from build123d import *

# Parameters (mm, degrees)
SKETCH2_W            = 125
SKETCH2_H            = 85
CREATE_BEAM_DEPTH    = 40
SKETCH3_W            = 119
SKETCH3_H            = 79
SKETCH3_R            = 7
REMOVE_OUTSIDE_DEPTH = 35
SKETCH4_R            = 7
LOWER_PILLARS_DEPTH  = 20


with BuildPart() as part:
    # Sketch2 → Create Beam (new body)
    with BuildSketch(Plane(origin=(0, 0, 0), x_dir=(1, 0, 0), z_dir=(0, 1, 0))):
        with Locations((62.5, 42.5)):
            Rectangle(SKETCH2_W, SKETCH2_H)
    extrude(amount=CREATE_BEAM_DEPTH)

    # Sketch3 → Remove Outside (cut)
    with BuildSketch(Plane(origin=(0, 40, 0), x_dir=(1, 0, 0), z_dir=(0, 1, 0))):
        with Locations((62.5, 42.5)):
            Rectangle(SKETCH3_W, SKETCH3_H)
        with Locations(Location((91, 33, 0), (0, 0, 270))):
            Circle(SKETCH3_R, mode=Mode.SUBTRACT)
        with Locations(Location((72, 33, 0), (0, 0, 270))):
            Circle(SKETCH3_R, mode=Mode.SUBTRACT)
        with Locations(Location((53, 33, 0), (0, 0, 270))):
            Circle(SKETCH3_R, mode=Mode.SUBTRACT)
        with Locations(Location((34, 33, 0), (0, 0, 270))):
            Circle(SKETCH3_R, mode=Mode.SUBTRACT)
        with Locations(Location((91, 52, 0), (0, 0, 270))):
            Circle(SKETCH3_R, mode=Mode.SUBTRACT)
        with Locations(Location((72, 52, 0), (0, 0, 270))):
            Circle(SKETCH3_R, mode=Mode.SUBTRACT)
        with Locations(Location((53, 52, 0), (0, 0, 270))):
            Circle(SKETCH3_R, mode=Mode.SUBTRACT)
        with Locations(Location((34, 52, 0), (0, 0, 270))):
            Circle(SKETCH3_R, mode=Mode.SUBTRACT)
    extrude(amount=-REMOVE_OUTSIDE_DEPTH, mode=Mode.SUBTRACT)

    # Sketch4 → Lower Pillars (cut)
    with BuildSketch(Plane(origin=(0, 40, 0), x_dir=(1, 0, 0), z_dir=(0, 1, 0))):
        with Locations(Location((34, 33, 0), (0, 0, 270))):
            Circle(SKETCH4_R)
        with Locations(Location((53, 33, 0), (0, 0, 270))):
            Circle(SKETCH4_R)
        with Locations(Location((91, 33, 0), (0, 0, 270))):
            Circle(SKETCH4_R)
        with Locations(Location((72, 33, 0), (0, 0, 270))):
            Circle(SKETCH4_R)
        with Locations(Location((91, 52, 0), (0, 0, 270))):
            Circle(SKETCH4_R)
        with Locations(Location((72, 52, 0), (0, 0, 270))):
            Circle(SKETCH4_R)
        with Locations(Location((53, 52, 0), (0, 0, 270))):
            Circle(SKETCH4_R)
        with Locations(Location((34, 52, 0), (0, 0, 270))):
            Circle(SKETCH4_R)
    extrude(amount=-LOWER_PILLARS_DEPTH, mode=Mode.SUBTRACT)


solid = part.part
The model under review builds one solid part; all positions refer to its coordinate system, in mm. A direction names the side the tool comes from. Give positions to 0.01 mm unless a question says otherwise; leave off trailing zeros. Order: outer loops, then holes, each group sorted by start corner. A loop starts at its lowest first (then second) coordinate and runs counter-clockwise, first axis right, second up. Notation, with made-up numbers: M 10,13 L 33,13 A16 ccw 33,19 Z; hole C 77.5,-22.5 d1. An arc over 180 degrees is marked long. Answer in a Markdown table with one row per item. Add a question column.
1. Add section B-B on y = 16. Count the separate pieces of the cut face and the enclosed holes in it, plus the area to 3 significant figures.
2. Add section D-D on z = -33. State the section outline as (x, y) points.
3. Add section C-C on x = 25. State the section outline as (y, z) points.
4. Machinability: for faces 4 (the cylindrical face through (58.902, 12.605, -48.237)), 5 (the flat face through (0, 20, -42)), which of the approach directions +Z, -Z, +X, -X, +Y, -Y give a long, thin tool a straight path to every point of the face, cutting with its end or side? Answer none if there is none.
5. Mouldability with a two-part tool opening along X and no side actions: class faces 1 (the cylindrical face through (58.902, 12.605, -29.237)), 2 (the flat face through (62, 20, -85)), 3 (the flat face through (125, 20, -42)) as released by +X, released by -X, zero draft, split by the parting line, or undercut.
6. For pin 1 Ø11 at (x, z) = (32, -54.5) entering from +Y; pin 2 Ø5 at (x, z) = (16, -10.5) entering from +Y, all flat-tipped, find the tip position at first contact; note any pin that passes through.
7. Add section A-A on y = 36.5. State the section outline as (x, z) points, plus the area to 3 significant figures.
8. To check wall thickness, follow line 1 along X through (y, z) = (6, -33.5); line 2 along X through (y, z) = (37.5, -62.5); line 3 along Z through (x, y) = (42, 6). State the ranges of each line that lie inside material, in increasing order.
The answers:
| question | item | result |
|---|---|---|
| 1 | separate pieces | 9 |
| 1 | enclosed holes | 1 |
| 1 | area | 2,460 mm2 |
| 2 | outline | M 0,0 L 125,0 L 125,40 L 122,40 L 122,5 L 98,5 L 98,20 L 84,20 L 84,5 L 79,5 L 79,20 L 65,20 L 65,5 L 60,5 L 60,20 L 46,20 L 46,5 L 41,5 L 41,20 L 27,20 L 27,5 L 3,5 L 3,40 L 0,40 Z |
| 3 | outline | M 0,-85 L 40,-85 L 40,-82 L 5,-82 L 5,-3 L 40,-3 L 40,0 L 0,0 Z |
| 4 | face 4 | +Y |
| 4 | face 5 | +Z, -Z, -X, +Y, -Y |
| 5 | face 1 | undercut |
| 5 | face 2 | zero draft |
| 5 | face 3 | released by +X |
| 6 | pin 1 | y = 20 |
| 6 | pin 2 | y = 5 |
| 7 | outline | M 0,-85 L 125,-85 L 125,0 L 0,0 Z; hole M 3,-82 L 122,-82 L 122,-3 L 3,-3 Z |
| 7 | area | 1,220 mm2 |
| 8 | line 1 | 0 to 3, 27.02 to 40.98, 46.02 to 59.98, 65.02 to 78.98, 84.02 to 97.98, 122 to 125 |
| 8 | line 2 | 0 to 3, 122 to 125 |
| 8 | line 3 | -85 to -82, -3 to 0 |
